```python
from build123d import *

# Parameters (mm, degrees)
SKETCH_1_R          = 12.5
SKETCH_1_R_2        = 10.7
EXTRUDE_1_DEPTH     = 190
SKETCH_3_W          = 12
SKETCH_3_H          = 4.814393821
CUT_EXTRUDE_1_DEPTH = 50


with BuildPart() as part:
    # Эскиз1 → Бобышка-Вытянуть1 (new body)
    with BuildSketch(Plane(origin=(0, 0, 0), x_dir=(1, 0, 0), z_dir=(0, 1, 0))):
        Circle(SKETCH_1_R)
        Circle(SKETCH_1_R_2, mode=Mode.SUBTRACT)
    extrude(amount=EXTRUDE_1_DEPTH)

    # Эскиз3 → Вырез-Вытянуть1 (cut)
    with BuildSketch(Plane(origin=(0, 190, 0), x_dir=(1, 0, 0), z_dir=(0, 1, 0))):
        with Locations((0, 10.407196911)):
            Rectangle(SKETCH_3_W, SKETCH_3_H)
    extrude(amount=-CUT_EXTRUDE_1_DEPTH, mode=Mode.SUBTRACT)


solid = part.part
```
The listing builds one solid part. Answer for the finished solid, in the listing's coordinates (mm). Coordinates: 2 decimals unless noted, no trailing zeros. Write each loop counter-clockwise with the first axis right and the second up, starting at its lowest first coordinate (ties: lowest second). Pieces come first, ordered by that corner, then holes. Notation, with made-up numbers: (47, 85) - (94, 85) arc R22 cw to (94, 118) - close; hole circle Ø11 at (-34.75, 47.5). An arc over 180 degrees is marked (long way). Return JSON: item names as keys, results as strings. Group by question number.
Q1. For a pull along X with two mould halves and no side action, classify faces 1 (the flat face through (-3.8, 190, 10.3)), 2 (the flat face through (0, 140, -11)), 3 (the cylindrical face through (5.77, 93.67, 11.09)) as +X half, -X half, draft (parallel to the pull), parting line (faces both ways), or undercut.
Q2. The part is cut by section B-B on z = 0. Write down the section's boundary in (x, y).
Q3. The part is cut by section C-C on y = 142. Write down the section's boundary in (x, z), and give its area (3 significant figures).
Q4. Find the intervals of material crossed by line 1 along Z through (x, y) = (0, 47); line 2 along Z through (x, y) = (0, 151.5), in increasing order. Write a range as [from, to].
Q5. The part is cut by section A-A on x = 0. Write down the section's boundary in (y, z).
Q6. The part is cut by section D-D on y = 49. Write down the section's boundary in (x, z), and give its area (3 significant figures).
Q7. Flat-ended cylindrical pins translate along their axes: pin 1 Ø3 at (x, y) = (-8.5, 31) entering from -Z; pin 2 Ø3 at (y, z) = (36, -7.5) entering from +X; pin 3 Ø4 at (x, z) = (-2, -10) entering from +Y. Find the tip coordinate at first contact, or state that the pin passes through.
Evaluation:
{
 "1": {"face 1": "draft", "face 2": "undercut", "face 3": "parting line"},
 "2": {"outline": "(-12.5, 0) - (-10.7, 0) - (-10.7, 190) - (-12.5, 190) - close; (10.7, 0) - (12.5, 0) - (12.5, 190) - (10.7, 190) - close"},
 "3": {"outline": "(-6, -10.97) - (-6, -8.86) arc R10.7 cw (long way) to (6, -8.86) - (6, -10.97) arc R12.5 ccw (long way) to start", "area": "108 mm2"},
 "4": {"line 1": "z = [-12.5, -10.7], [10.7, 12.5]", "line 2": "z = [10.7, 12.5]"},
 "5": {"outline": "(0, -12.5) - (140, -12.5) - (140, -10.7) - (0, -10.7) - close; (0, 10.7) - (190, 10.7) - (190, 12.5) - (0, 12.5) - close"},
 "6": {"outline": "circle Ø25 at (0, 0); hole circle Ø21.4 at (0, 0)", "area": "131 mm2"},
 "7": {"pin 1": "stops at z = -10.36", "pin 2": "stops at x = 10.97", "pin 3": "stops at y = 140"}
}
